from build123d import *

# Parameters (mm, degrees)
F0_R     = 20
F1_DEPTH = 12.7
F2_R     = 6.477
F3_DEPTH = 50.801
F4_DEPTH = 25.4


with BuildPart() as f1:
    # F0 (on Front) → F1 (new body, symmetric)
    with BuildSketch(Plane.XZ):
        with BuildLine():
            ThreePointArc((-38.1, 17.78), (-36.210287, 0.987833), (-30.635678, -14.964333))
            ThreePointArc((-30.635678, -14.964333), (0, -34.095103), (30.635678, -14.964333))
            ThreePointArc((30.635678, -14.964333), (36.210287, 0.987833), (38.1, 17.78))
            Line((38.1, 17.78), (38.1, 25.4))
            Line((38.1, 25.4), (12.7, 25.4))
            Line((12.7, 25.4), (12.7, 50.8))
            Line((12.7, 50.8), (-12.7, 50.8))
            Line((-12.7, 50.8), (-12.7, 25.4))
            Line((-12.7, 25.4), (-38.1, 25.4))
            Line((-38.1, 25.4), (-38.1, 17.78))
        make_face()
        Circle(F0_R, mode=Mode.SUBTRACT)
    extrude(amount=F1_DEPTH, both=True)

    # F2 (on face) → F3 (cut, through all)
    with BuildSketch(Plane(origin=(-12.7, 0, 0), x_dir=(0, -1, 0), z_dir=(-1, 0, 0))):
        with Locations((0, 38.1)):
            Circle(F2_R)
    extrude(amount=-F3_DEPTH, mode=Mode.SUBTRACT)

    # F2 (on face) → F4 (join)
    with BuildSketch(Plane(origin=(-12.7, 0, 0), x_dir=(0, -1, 0), z_dir=(-1, 0, 0))):
        with BuildLine():
            Line((-12.7, 50.8), (12.7, 50.8))
            ThreePointArc((12.7, 50.8), (0, 63.5), (-12.7, 50.8))
        make_face()
    extrude(amount=-F4_DEPTH)


solid = f1.part
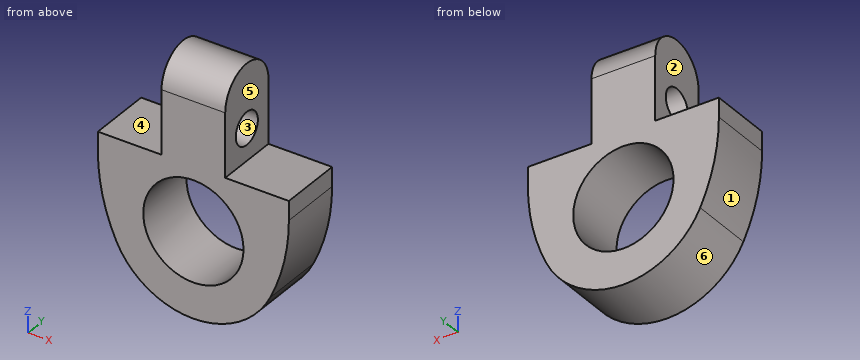
The model under review builds one solid part; all positions refer to its coordinate system, in mm. Face numbers are marked on the shaded views. A direction names the side the tool comes from. Give positions to 0.01 mm unless a question says otherwise; leave off trailing zeros. Write each loop counter-clockwise with the first axis right and the second up, starting at its lowest first coordinate (ties: lowest second). Pieces come first, ordered by that corner, then holes. Notation, with made-up numbers: M 45,87 L 79,87 A11 cw 79,106 Z; hole C 83,33 d1. An arc over 180 degrees is marked long. One line per question, with ' | ' between items. Start each with the question number.
Item 1: We need section B-B on x = 0. Write out the cut boundary in (y, z).
Item 2: For pin 1 (3 mm diameter, centred on x = -30, y = 7.5, fed in from +Z); pin 2 (12.5 mm diameter, centred on y = 1, z = 53, fed in from +X); pin 3 (1 mm diameter, centred on x = 2.5, y = 1, fed in from -Z); pin 4 (2 mm diameter, centred on x = -18.5, z = 3, fed in from +Y), all flat-tipped, find the tip position at first contact; note any pin that passes through.
Item 3: We need section C-C on z = 38.1. Write out the cut boundary in (x, y).
Item 4: We need section A-A on y = 0. Write out the cut boundary in (x, z), plus the area to 3 significant figures.
Item 5: We need section D-D on x = 16.5. Write out the cut boundary in (y, z).
Item 6: Wall thickness on line 1 (Y direction, x = -6, z = 38); line 2 (Z direction, x = -9, y = -1.5); line 3 (Z direction, x = 5.5, y = -5.5): over which ranges is each line inside the solid? List them lowest first. Write a range as from..to.
Item 7: For the marked faces 4, 5 and 6, list the 3-axis set-ups (+Z, -Z, +X, -X, +Y, -Y) from which the entire face can be reached by the end or side of a thin tool; tool diameter is ignored.
Item 8: Draft analysis for pull direction Z (two halves, no side actions). For the marked faces 1, 2 and 3, state which applies: released by +Z, released by -Z, zero draft, split by the parting line, or undercut.
Results found:
1) outline: M -12.7,-34.1 L 12.7,-34.1 L 12.7,-20 L -12.7,-20 Z; M -12.7,20 L 12.7,20 L 12.7,50.8 A12.7 ccw -12.7,50.8 Z; hole C 0,38.1 d12.95
2) pin 1: stops at z = 25.4 | pin 2: stops at x = 12.7 | pin 3: stops at z = -34.04 | pin 4: passes through
3) outline: M -12.7,-12.7 L 12.7,-12.7 L 12.7,-6.48 L -12.7,-6.48 Z; M -12.7,6.48 L 12.7,6.48 L 12.7,12.7 L -12.7,12.7 Z
4) outline: M -38.1,17.78 A75.55 ccw -30.64,-14.96 A34.1 ccw 30.64,-14.96 A75.55 ccw 38.1,17.78 L 38.1,25.4 L 12.7,25.4 L 12.7,31.62 L -12.7,31.62 L -12.7,25.4 L -38.1,25.4 Z; M -12.7,44.58 L 12.7,44.58 L 12.7,63.5 L -12.7,63.5 Z; hole C 0,0 d40 | area: 3,140 mm2
5) outline: M -12.7,-29.84 L 12.7,-29.84 L 12.7,-11.3 L -12.7,-11.3 Z; M -12.7,11.3 L 12.7,11.3 L 12.7,25.4 L -12.7,25.4 Z
6) line 1: y = -12.7..-6.48, 6.48..12.7 | line 2: z = -32.89..-17.86, 17.86..31.8, 44.4..63.41 | line 3: z = -33.65..-19.23, 19.23..34.68, 41.52..62.25
7) face 4: +Z, -X, +Y, -Y | face 5: +Z, +X, +Y, -Y | face 6: -Z, +Y, -Y
8) face 1: released by -Z | face 2: zero draft | face 3: undercut
